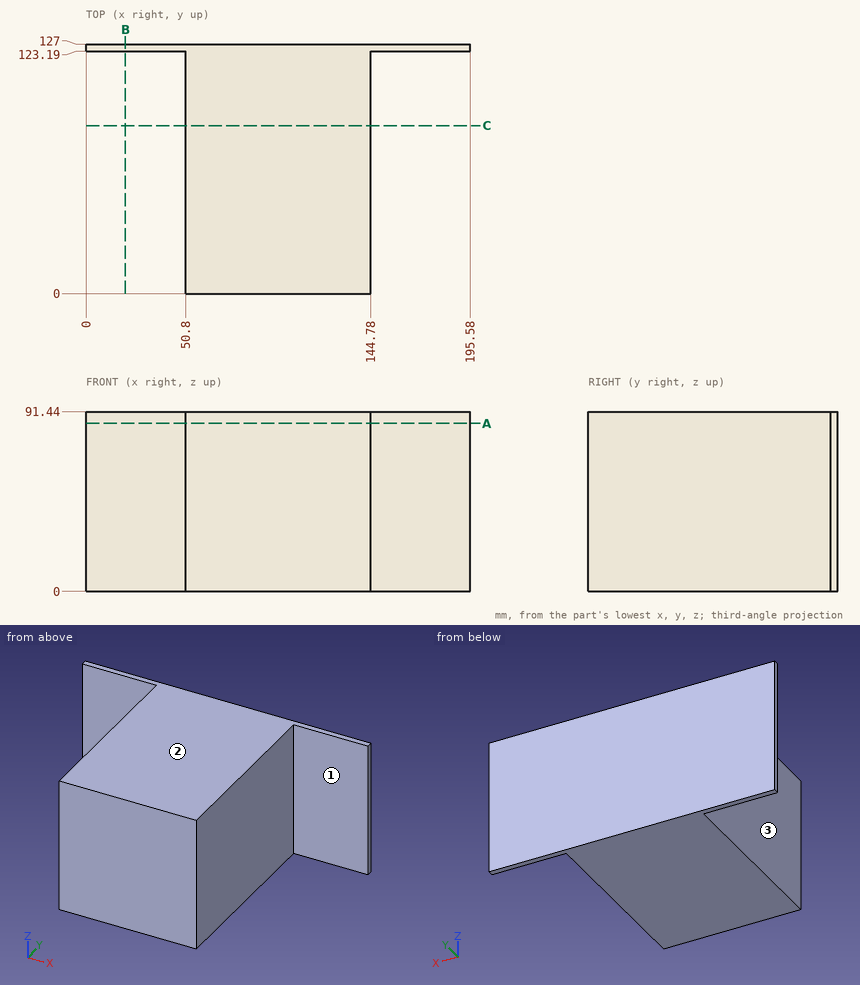
For this review, use the dimensioned drawing (mm, ordinates from the lowest corner) and the shaded views. A direction names the side the tool comes from. Coordinates: 2 decimals unless noted, no trailing zeros. Loops run counter-clockwise (first coordinate to the right, second up) from the corner with the lowest first, then second, coordinate; pieces in that order, holes last.
1. For line 1 (X direction, y = 20, z = 39); line 2 (Y direction, x = 159, z = 27.5), list the stretches that pass through material, from the lowest coordinate up.
2. For the marked faces 1, 2 and 3, list the 3-axis set-ups (+Z, -Z, +X, -X, +Y, -Y) from which the entire face can be reached by the end or side of a thin tool; tool diameter is ignored.
3. Add section A-A, the plane z = 85.5. Give the boundary of the cut face in (x, y), then the cut area to 3 significant figures.
4. Add section C-C, the plane y = 85.5. Give the boundary of the cut face in (x, z).
5. Insertion check: P1, Ø4, axis at y = 24, z = 46.5, coming from the +X side; P2, Ø8, axis at x = 95.5, y = 24, coming from the -Z side; P3, Ø10, axis at y = 75.5, z = 32, coming from the -X side. Each pin has a flat end and moves straight along its axis. Give the tip position at first contact, or say it passes through.
6. Add section B-B, the plane x = 20. Give the boundary of the cut face in (y, z), then the cut area to 3 significant figures.
Result:
1. line 1: x = 50.8 to 144.78
1. line 2: y = 123.19 to 127
2. face 1: +Z, -Z, +X, -Y
2. face 2: +Z, +X, -X, +Y, -Y
2. face 3: +Z, -Z, -X, -Y
3. outline: (0, 123.19) - (50.8, 123.19) - (50.8, 0) - (144.78, 0) - (144.78, 123.19) - (195.58, 123.19) - (195.58, 127) - (0, 127) - close
3. area: 12,300 mm2
4. outline: (50.8, 0) - (144.78, 0) - (144.78, 91.44) - (50.8, 91.44) - close
5. P1: stops at x = 144.78
5. P2: stops at z = 0
5. P3: stops at x = 50.8
6. outline: (123.19, 0) - (127, 0) - (127, 91.44) - (123.19, 91.44) - close
6. area: 348 mm2
